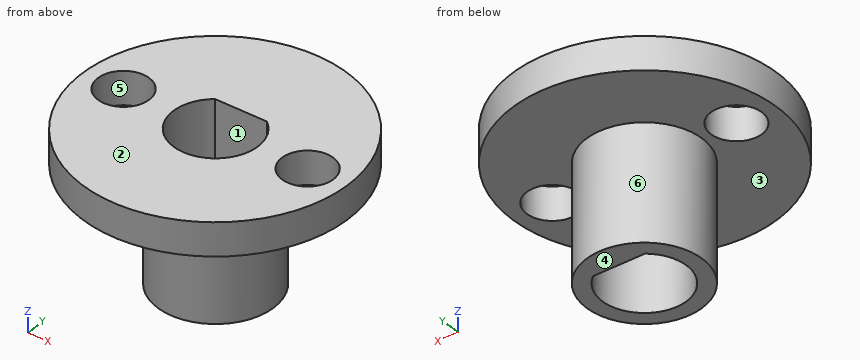
```python
from build123d import *

# Parameters (mm, degrees)
EXTRUDE_1_DEPTH          = 6
EXTRUDE_1_DEPTH_BACK     = 3
SKETCH_1_R               = 3.5
CUT_EXTRUDE_1_DEPTH      = 11.271319292
CUT_EXTRUDE_1_DEPTH_BACK = 11.271319292
SKETCH_3_R               = 8
EXTRUDE_2_DEPTH          = 2
CUT_EXTRUDE_2_DEPTH      = 15.480802494
SKETCH_5_R               = 1.55
CUT_EXTRUDE_3_DEPTH      = 2.5


with BuildPart() as part:
    # 草图1 → 凸台-拉伸1 (new, two sides: drawn at the far end of the back side and taken through both)
    with BuildSketch(Plane.XY.offset(-EXTRUDE_1_DEPTH_BACK)):
        Circle(SKETCH_1_R)
    extrude(amount=EXTRUDE_1_DEPTH + EXTRUDE_1_DEPTH_BACK)

    # 草图2 → 切除-拉伸1 (cut, two sides: drawn at the far end of the back side and taken through both)
    with BuildSketch(Plane(origin=(0, 0, -3), x_dir=(-1, 0, 0), z_dir=(0, 0, -1)).offset(-CUT_EXTRUDE_1_DEPTH_BACK)):
        with BuildLine():
            Line((1.581929202, 2), (-1.581929202, 2))
            ThreePointArc((-1.581929202, 2), (0, -2.55), (1.581929202, 2))
        make_face()
    extrude(amount=CUT_EXTRUDE_1_DEPTH + CUT_EXTRUDE_1_DEPTH_BACK, mode=Mode.SUBTRACT)

    # 草图3 → 凸台-拉伸2 (add)
    with BuildSketch(Plane.XY.offset(6)):
        with Locations((0, -0.043235721)):
            Circle(SKETCH_3_R)
    extrude(amount=-EXTRUDE_2_DEPTH)

    # 草图4 → 切除-拉伸2 (cut, through all)
    with BuildSketch(Plane.XY.offset(6)):
        with BuildLine():
            Line((-1.581929202, 2), (1.581929202, 2))
            ThreePointArc((1.581929202, 2), (0, -2.55), (-1.581929202, 2))
        make_face()
    extrude(amount=-CUT_EXTRUDE_2_DEPTH, mode=Mode.SUBTRACT)

    # 草图5 → 切除-拉伸3 (cut)
    with BuildSketch(Plane.XY.offset(6)):
        with Locations((5.6, 0)):
            Circle(SKETCH_5_R)
        with Locations((-5.6, 0)):
            Circle(SKETCH_5_R)
    extrude(amount=-CUT_EXTRUDE_3_DEPTH, mode=Mode.SUBTRACT)


solid = part.part
```
Geometry check sheet. Reference: the model listing, model coordinates, mm. Face numbers are marked on the shaded views. A direction names the side the tool comes from. Coordinates: 2 decimals unless noted, no trailing zeros. Loops run counter-clockwise (first coordinate to the right, second up) from the corner with the lowest first, then second, coordinate; pieces in that order, holes last.
Item 1: Sectioned sample at B-B, the plane z = 1.5. Record the boundary of the cut face in (x, y).
Item 2: Thickness scan on line 1 (X direction, y = 0, z = -1); line 2 (Y direction, x = 0, z = 1.5); line 3 (Z direction, x = 3.5, y = -1). Record the ranges inside material, lowest first.
Item 3: Access from +Z, -Z, +X, -X, +Y, -Y to the whole of each face (thin tool, end or side, straight path). Record for the marked faces 1, 2 and 3.
Item 4: Sectioned sample at D-D, the plane z = 4.25. Record the boundary of the cut face in (x, y).
Item 5: Sectioned sample at A-A, the plane x = 0. Record the boundary of the cut face in (y, z), then the cut area to 4 significant figures.
Item 6: Go/stop test with flat-tipped pins: pin 1 Ø6 at (x, y) = (1, -1.5) entering from -Z; pin 2 Ø2 at (x, z) = (-5.5, 0) entering from +Y; pin 3 Ø1.6 at (x, z) = (0.5, 2) entering from -Y. Record where each tip stops, or that it passes through.
Item 7: Sectioned sample at C-C, the plane x = -5.6. Record the boundary of the cut face in (y, z).
Item 8: Release check for a two-part mould opening along Y. For the marked faces 4, 5 and 6 record: released by +Y, released by -Y, zero draft, split by the parting line, or undercut.
Check result:
1. outline: circle Ø7 at (0, 0); hole (-1.58, 2) arc R2.55 ccw (long way) to (1.58, 2) - close
2. line 1: x = -3.5 to -2.55, 2.55 to 3.5
2. line 2: y = -3.5 to -2.55, 2 to 3.5
2. line 3: z = 4 to 6
3. face 1: +Z, -Z
3. face 2: +Z, +X, -X, +Y, -Y
3. face 3: -Z
4. outline: circle Ø16 at (0, -0.04); hole circle Ø3.1 at (-5.6, 0); hole (-1.58, 2) arc R2.55 ccw (long way) to (1.58, 2) - close; hole circle Ø3.1 at (5.6, 0)
5. outline: (-8.04, 4) - (-3.5, 4) - (-3.5, -3) - (-2.55, -3) - (-2.55, 6) - (-8.04, 6) - close; (2, -3) - (3.5, -3) - (3.5, 4) - (7.96, 4) - (7.96, 6) - (2, 6) - close
5. area: 40.05 mm2
6. pin 1: stops at z = -3
6. pin 2: passes through
6. pin 3: stops at y = -3.5
7. outline: (-5.76, 4) - (-1.55, 4) - (-1.55, 6) - (-5.76, 6) - close; (1.55, 4) - (5.67, 4) - (5.67, 6) - (1.55, 6) - close
8. face 4: zero draft
8. face 5: undercut
8. face 6: split by the parting line
